Part model, mm, in its own coordinate system. Face numbers are marked on the shaded views. A direction names the side the tool comes from. Coordinates: 2 decimals unless noted, no trailing zeros. Loops run counter-clockwise (first coordinate to the right, second up) from the corner with the lowest first, then second, coordinate; pieces in that order, holes last. Notation, with made-up numbers: M 42,55.5 L 74,55.5 A18 ccw 74,64.5 Z; hole C -34,-25.75 d5. An arc over 180 degrees is marked long. Answer as a JSON object with one key per item and string values. Group by question number.
1. Saw through at B-B on y = 1.65. Write the cut outline in (x, z) (1 decimal), then the cut area to 3 significant figures.
2. Saw through at A-A on z = 0. Write the cut outline in (x, y).
3. Mould opens along X. For the marked faces 1, 2 and 3 say: released by +X, released by -X, zero draft, split by the parting line, or undercut.
4. Saw through at C-C on x = 1. Write the cut outline in (y, z), then the cut area to 3 significant figures.
5. Drill centre lines: L1, parallel to X at y = 2.2, z = 0; L2, parallel to X at y = 0.65, z = -1; L3, parallel to X at y = 1.45, z = 13 (3 decimals). Where is each one in solid material? Low to high.
6. 3-axis set-ups, long thin cutter, end or side, ignore diameter. For the marked faces 4 and 5: which of +Z, -Z, +X, -X, +Y, -Y reach the whole face in a straight line?
7. Saw through at D-D on z = 13.5. Write the cut outline in (x, y) (3 decimals), then the cut area to 3 significant figures.
8. Drop flat-ended pins along their axis: pin 1 Ø0.9 at (y, z) = (1, 12) entering from +X; pin 2 Ø1.4 at (y, z) = (1.5, 0.5) entering from -X; pin 3 Ø1.4 at (y, z) = (1, 0.5) entering from +X; pin 4 Ø1.4 at (x, y) = (0.5, 1.5) entering from -Z. Give the stop position or say it passes through.
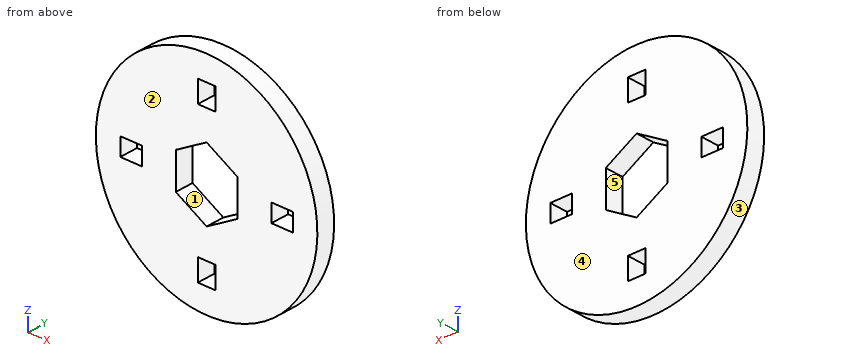
from build123d import *

# Parameters (mm, degrees)
SKETCH1_R           = 17.962739212
SKETCH1_W           = 3.5
SKETCH1_H           = 2.85
SKETCH1_W_2         = 2.85
SKETCH1_H_2         = 3.5
BOSS_EXTRUDE1_DEPTH = 3


with BuildPart() as part:
    # Sketch1 → Boss-Extrude1 (new body)
    with BuildSketch(Plane(origin=(0, 0, 0), x_dir=(1, 0, 0), z_dir=(0, 1, 0))):
        with Locations(Location((0, 0, 0), (0, 0, 270))):
            Circle(SKETCH1_R)
        with Locations((-12.25, 0)):
            Rectangle(SKETCH1_W, SKETCH1_H, mode=Mode.SUBTRACT)
        with Locations((0, -12.25)):
            Rectangle(SKETCH1_W_2, SKETCH1_H_2, mode=Mode.SUBTRACT)
        with Locations((0, 12.25)):
            Rectangle(SKETCH1_W_2, SKETCH1_H_2, mode=Mode.SUBTRACT)
        with Locations((12.25, 0)):
            Rectangle(SKETCH1_W, SKETCH1_H, mode=Mode.SUBTRACT)
        Polygon((0, -5.773502692), (5, -2.886751346), (5, 2.886751346), (0, 5.773502692), (-5, 2.886751346), (-5, -2.886751346), align=None, mode=Mode.SUBTRACT)
    extrude(amount=BOSS_EXTRUDE1_DEPTH)


solid = part.part
Outcome:
{
 "1": {"outline": "C 0,0 d35.9; hole M -14,-1.4 L -10.5,-1.4 L -10.5,1.4 L -14,1.4 Z; hole M -5,-2.9 L 0,-5.8 L 5,-2.9 L 5,2.9 L 0,5.8 L -5,2.9 Z; hole M -1.4,-14 L 1.4,-14 L 1.4,-10.5 L -1.4,-10.5 Z; hole M -1.4,10.5 L 1.4,10.5 L 1.4,14 L -1.4,14 Z; hole M 10.5,-1.4 L 14,-1.4 L 14,1.4 L 10.5,1.4 Z", "area": "887 mm²"},
 "2": {"outline": "M -17.96,0 L -14,0 L -14,3 L -17.96,3 Z; M -10.5,0 L -5,0 L -5,3 L -10.5,3 Z; M 5,0 L 10.5,0 L 10.5,3 L 5,3 Z; M 14,0 L 17.96,0 L 17.96,3 L 14,3 Z"},
 "3": {"face 1": "undercut", "face 2": "zero draft", "face 3": "split by the parting line"},
 "4": {"outline": "M 0,-17.93 L 3,-17.93 L 3,-14 L 0,-14 Z; M 0,-10.5 L 3,-10.5 L 3,-5.2 L 0,-5.2 Z; M 0,5.2 L 3,5.2 L 3,10.5 L 0,10.5 Z; M 0,14 L 3,14 L 3,17.93 L 0,17.93 Z", "area": "55.4 mm²"},
 "5": {"L1": "x = -17.96 to -14, -10.5 to -5, 5 to 10.5, 14 to 17.96", "L2": "x = -17.93 to -14, -10.5 to -5, 5 to 10.5, 14 to 17.93", "L3": "x = -12.396 to -1.425, 1.425 to 12.396"},
 "6": {"face 4": "+Z, -Z, +X, -X, +Y", "face 5": "+Y, -Y"},
 "7": {"outline": "M -11.849,0 L -1.425,0 L -1.425,3 L -11.849,3 Z; M 1.425,0 L 11.849,0 L 11.849,3 L 1.425,3 Z", "area": "62.5 mm²"},
 "8": {"pin 1": "stops at x = 13.76", "pin 2": "stops at x = -17.96", "pin 3": "stops at x = 17.96", "pin 4": "stops at z = -17.96"}
}
